The listing builds one solid part. Answer for the finished solid, in the listing's coordinates (mm). Face numbers are marked on the shaded views. Coordinates: 2 decimals unless noted, no trailing zeros. Write each loop counter-clockwise with the first axis right and the second up, starting at its lowest first coordinate (ties: lowest second). Pieces come first, ordered by that corner, then holes.
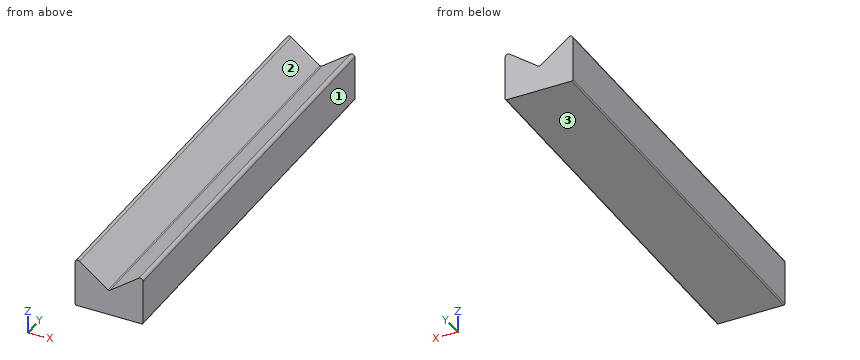
from build123d import *

# Parameters (mm, degrees)
F1_DEPTH = 38.1
F2_R     = 0.254
F3_R     = 0.127


with BuildPart() as f1:
    # F0 (on Front) → F1 (new body)
    with BuildSketch(Plane.XZ):
        Polygon((3.175, -2.38125), (0, -2.38125), (0, -4.7625), (6.35, -4.7625), (6.35, -2.38125), align=None)
        Polygon((3.175, -2.38125), (0, 0), (0, -2.38125), align=None)
        Polygon((6.35, -2.38125), (6.35, 0), (3.175, -2.38125), align=None)
    extrude(amount=F1_DEPTH)

    # F2
    f2_edges = [f1.edges().sort_by_distance(p)[0] for p in [
        (0, -19.05, 0),
        (6.35, -19.05, 0),
    ]]
    fillet(f2_edges, radius=F2_R)

    # F3
    f3_edges = [f1.edges().sort_by_distance(p)[0] for p in [
        (3.175, -19.05, -2.38125),
        (6.35, -19.05, -4.7625),
        (0, -19.05, -4.7625),
    ]]
    fillet(f3_edges, radius=F3_R)


solid = f1.part
1. Section D-D on x = 4.75 is taken. Give the vertices of the cut face in (y, z).
Results found:
outline: (-38.1, -4.76) - (0, -4.76) - (0, -1.2) - (-38.1, -1.2) - close
2. Section C-C on x = 1 is taken. Give the vertices of the cut face in (y, z), then the cut area to 3 significant figures.
Results found:
outline: (-38.1, -4.76) - (0, -4.76) - (0, -0.75) - (-38.1, -0.75) - close
area: 153 mm2
3. Find the intervals of material crossed by L1, parallel to X at y = -8, z = -1.6; L2, parallel to X at y = -26.5, z = -0.8; L3, parallel to Z at x = 0.5, y = -14 (1 decimal), in increasing order.
Results found:
L1: x = 0 to 2.13, 4.22 to 6.35
L2: x = 0 to 1.07, 5.28 to 6.35
L3: z = -4.8 to -0.4
4. Section B-B on z = -1.6 is taken. Give the vertices of the cut face in (x, y).
Results found:
outline: (0, -38.1) - (2.13, -38.1) - (2.13, 0) - (0, 0) - close; (4.22, -38.1) - (6.35, -38.1) - (6.35, 0) - (4.22, 0) - close
5. For a pull along X with two mould halves and no side action, classify the marked faces 1, 2 and 3 as pulls with the +X half, pulls with the -X half, needs draft (parallel to the pull), parting line crosses it, or undercut.
Results found:
face 1: pulls with the +X half
face 2: undercut
face 3: needs draft
